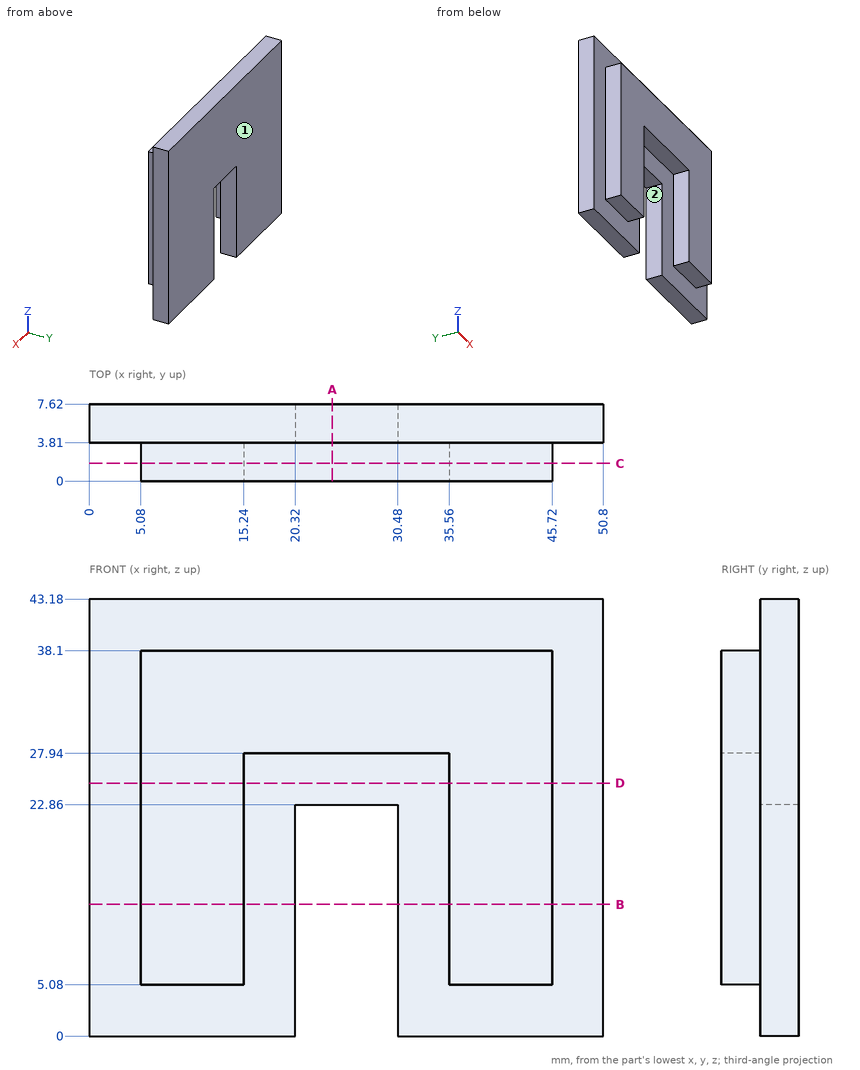
Check sheet for the drawn part. Datum: minimum x, y, z corner. Units: mm. A direction names the side the tool comes from. Round coordinates to 2 decimals unless told otherwise and drop trailing zeros. Order: outer loops, then holes, each group sorted by start corner. A loop starts at its lowest first (then second) coordinate and runs counter-clockwise, first axis right, second up.
(1) Go/stop test with flat-tipped pins: P1, Ø4, axis at x = 37.5, z = 36, coming from the -Y side; P2, Ø1.1, axis at x = 42, y = 1.5, coming from the -Z side; P3, Ø1.9, axis at y = 2, z = 27.5, coming from the -X side; P4, Ø4, axis at x = 25, y = 2, coming from the -Z side. Record where each tip stops, or that it passes through.
(2) Cross-section at A-A, the plane x = 24. Enter the section's corners in (y, z).
(3) Cross-section at C-C, the plane y = 1.75. Enter the section's corners in (x, z), and give its area (3 significant figures).
(4) Cross-section at B-B, the plane z = 13. Enter the section's corners in (x, y), and give its area (3 significant figures).
(5) Cross-section at D-D, the plane z = 25. Enter the section's corners in (x, y), and give its area (3 significant figures).
(6) Scan lines: probe 1 along X at (y, z) = (5, 9); probe 2 along X at (y, z) = (1, 7.5); probe 3 along Z at (x, y) = (43, 2). Record each from-to range of solid material in increasing order.
(7) Access from +Z, -Z, +X, -X, +Y, -Y to the whole of each face (thin tool, end or side, straight path). Record for the marked faces 1 and 2.
Check sheet entries:
1. P1: stops at y = 0
1. P2: stops at z = 5.08
1. P3: stops at x = 5.08
1. P4: stops at z = 22.86
2. outline: (0, 27.94) - (3.81, 27.94) - (3.81, 22.86) - (7.62, 22.86) - (7.62, 43.18) - (3.81, 43.18) - (3.81, 38.1) - (0, 38.1) - close
3. outline: (5.08, 5.08) - (15.24, 5.08) - (15.24, 27.94) - (35.56, 27.94) - (35.56, 5.08) - (45.72, 5.08) - (45.72, 38.1) - (5.08, 38.1) - close
3. area: 877 mm2
4. outline: (0, 3.81) - (5.08, 3.81) - (5.08, 0) - (15.24, 0) - (15.24, 3.81) - (20.32, 3.81) - (20.32, 7.62) - (0, 7.62) - close; (30.48, 3.81) - (35.56, 3.81) - (35.56, 0) - (45.72, 0) - (45.72, 3.81) - (50.8, 3.81) - (50.8, 7.62) - (30.48, 7.62) - close
4. area: 232 mm2
5. outline: (0, 3.81) - (5.08, 3.81) - (5.08, 0) - (15.24, 0) - (15.24, 3.81) - (35.56, 3.81) - (35.56, 0) - (45.72, 0) - (45.72, 3.81) - (50.8, 3.81) - (50.8, 7.62) - (0, 7.62) - close
5. area: 271 mm2
6. probe 1: x = 0 to 20.32, 30.48 to 50.8
6. probe 2: x = 5.08 to 15.24, 35.56 to 45.72
6. probe 3: z = 5.08 to 38.1
7. face 1: +Z, -Z, +X, -X, +Y
7. face 2: -Z, +Y, -Y
